Check sheet for the modelled part. Datum: model origin and axes. Units: mm. Face numbers are marked on the shaded views. Round coordinates to 2 decimals unless told otherwise and drop trailing zeros. Write each loop counter-clockwise with the first axis right and the second up, starting at its lowest first coordinate (ties: lowest second). Pieces come first, ordered by that corner, then holes.
Item 1: Material ranges on line 1 along X through (y, z) = (50.8, 11.75) (3 decimals); line 2 along Y through (x, z) = (1, 10.25); line 3 along X through (y, z) = (50, 2.25) (3 decimals), recorded low to high.
Item 2: Section check B-B, the plane x = 46. Record the cut outline in (y, z).
Item 3: Depth check by flat-ended pin: pin 1 (4 mm diameter, centred on y = -44.5, z = 3, fed in from -X); pin 2 (2 mm diameter, centred on x = 36, z = 6, fed in from +Y) (3 decimals); pin 3 (12 mm diameter, centred on y = 26, z = 4, fed in from -X); pin 4 (5.5 mm diameter, centred on x = 0, y = -63.5, fed in from +Z). Enter the tip coordinate at first touch or a pass-through.
Item 4: Section check D-D, the plane y = -38. Record the cut outline in (x, z) (3 decimals).
Item 5: Section check C-C, the plane x = 23. Record the cut outline in (y, z), plus the area to 3 significant figures.
Item 6: Section check A-A, the plane z = 19.5. State how many separate pieces and enclosed holes the cut face has, plus the area to 3 significant figures.
Item 7: Release check for a two-part mould opening along Y. For the marked faces 1, 2 and 3 record: pulls with the +Y half, pulls with the -Y half, needs draft (parallel to the pull), parting line crosses it, or undercut.
from build123d import *

# Parameters (mm, degrees)
F0_R     = 3.175
F1_DEPTH = 25.4


with BuildPart() as f1:
    # F0 (on Top) → F1 (new body)
    with BuildSketch(Plane.XY):
        with BuildLine():
            ThreePointArc((-9.525, 50.8), (-6.7351920908, 44.0648079092), (0, 41.275))
            ThreePointArc((0, 41.275), (6.7351920908, 44.0648079092), (9.525, 50.8))
            ThreePointArc((9.525, 50.8), (0, 60.325), (-9.525, 50.8))
        make_face()
        with BuildLine():
            ThreePointArc((3.175, 50.8), (2.2450640303, 48.5549359697), (0, 47.625))
            ThreePointArc((0, 47.625), (-2.2450640303, 53.0450640303), (3.175, 50.8))
        make_face(mode=Mode.SUBTRACT)
        with BuildLine():
            ThreePointArc((9.525, 50.8), (6.7351920908, 44.0648079092), (0, 41.275))
            Line((0, 41.275), (0, 36.5252))
            Line((0, 36.5252), (0, 15.875))
            ThreePointArc((0, 15.875), (9.7463072395, 12.5309664508), (15.3865384615, 3.9076923077))
            Line((15.3865384615, 3.9076923077), (9.525, 50.8))
        make_face()
        with BuildLine():
            Line((0, 36.5252), (0, 41.275))
            ThreePointArc((0, 41.275), (-6.7351920908, 44.0648079092), (-9.525, 50.8))
            Line((-9.525, 50.8), (-15.7474568951, 2.0082894055))
            ThreePointArc((-15.7474568951, 2.0082894055), (-10.4912828264, 11.9142188018), (0, 15.875))
            Line((0, 15.875), (0, 36.5252))
        make_face()
        with Locations((-3.175, 36.5252)):
            Circle(F0_R, mode=Mode.SUBTRACT)
        with BuildLine():
            ThreePointArc((15.3865384615, 3.9076923077), (9.7463072395, 12.5309664508), (0, 15.875))
            Line((0, 15.875), (0, 3.175))
            ThreePointArc((0, 3.175), (2.2450640303, 2.2450640303), (3.175, 0))
            ThreePointArc((3.175, 0), (2.2450640303, -2.2450640303), (0, -3.175))
            Line((0, -3.175), (0, -15.875))
            ThreePointArc((0, -15.875), (10.0526499203, -12.2865721249), (15.5606435644, -3.1435643564))
            Line((15.5606435644, -3.1435643564), (15.875, 0))
            Line((15.875, 0), (15.3865384615, 3.9076923077))
        make_face()
        with BuildLine():
            Line((0, 3.175), (0, 15.875))
            ThreePointArc((0, 15.875), (-10.4912828264, 11.9142188018), (-15.7474568951, 2.0082894055))
            ThreePointArc((-15.7474568951, 2.0082894055), (-11.9142188018, -10.4912828264), (0, -15.875))
            Line((0, -15.875), (0, -3.175))
            ThreePointArc((0, -3.175), (-3.175, 0), (0, 3.175))
        make_face()
        with BuildLine():
            ThreePointArc((0, -15.875), (-11.9142188018, -10.4912828264), (-15.7474568951, 2.0082894055))
            Line((-15.7474568951, 2.0082894055), (-16.0035761028, 0))
            Line((-16.0035761028, 0), (-9.525, -63.5))
            ThreePointArc((-9.525, -63.5), (-6.7351920908, -56.7648079092), (0, -53.975))
            Line((0, -53.975), (0, -15.875))
        make_face()
        with BuildLine():
            ThreePointArc((15.875, 0), (15.7524112928, 1.9690514116), (15.3865384615, 3.9076923077))
            Line((15.3865384615, 3.9076923077), (15.875, 0))
        make_face()
        with BuildLine():
            ThreePointArc((15.5606435644, -3.1435643564), (10.0526499203, -12.2865721249), (0, -15.875))
            Line((0, -15.875), (0, -53.975))
            Line((0, -53.975), (0.6794904459, -53.9992675159))
            ThreePointArc((0.6794904459, -53.9992675159), (6.9712901065, -57.0094885216), (9.525, -63.5))
            Line((9.525, -63.5), (36.5125, -63.5))
            ThreePointArc((36.5125, -63.5), (38.8373399243, -57.8873399243), (44.45, -55.5625))
            Line((44.45, -55.5625), (14.6753932646, -54.499121188))
            ThreePointArc((14.6753932646, -54.499121188), (11.8227843813, -53.1408361956), (10.8618983328, -50.1310166722))
            Line((10.8618983328, -50.1310166722), (15.5606435644, -3.1435643564))
        make_face()
        with BuildLine():
            ThreePointArc((15.5606435644, -3.1435643564), (15.7962153946, -1.5796215395), (15.875, 0))
            Line((15.875, 0), (15.5606435644, -3.1435643564))
        make_face()
        with BuildLine():
            Line((0, -60.325), (0, -53.975))
            ThreePointArc((0, -53.975), (-6.7351920908, -56.7648079092), (-9.525, -63.5))
            ThreePointArc((-9.525, -63.5), (-6.7351920908, -70.2351920908), (0, -73.025))
            Line((0, -73.025), (0.6794904459, -73.0007324841))
            ThreePointArc((0.6794904459, -73.0007324841), (6.9712901065, -69.9905114784), (9.525, -63.5))
            Line((9.525, -63.5), (3.175, -63.5))
            ThreePointArc((3.175, -63.5), (-2.2450640303, -65.7450640303), (0, -60.325))
        make_face()
        with BuildLine():
            Line((0.6794904459, -73.0007324841), (0, -73.025))
            ThreePointArc((0, -73.025), (0.3399618281, -73.0189311877), (0.6794904459, -73.0007324841))
        make_face()
        with BuildLine():
            Line((36.5125, -63.5), (9.525, -63.5))
            ThreePointArc((9.525, -63.5), (6.9712901065, -69.9905114784), (0.6794904459, -73.0007324841))
            Line((0.6794904459, -73.0007324841), (44.45, -71.4375))
            ThreePointArc((44.45, -71.4375), (38.8373399243, -69.1126600757), (36.5125, -63.5))
        make_face()
        with BuildLine():
            ThreePointArc((44.45, -55.5625), (38.8373399243, -57.8873399243), (36.5125, -63.5))
            Line((36.5125, -63.5), (41.275, -63.5))
            ThreePointArc((41.275, -63.5), (42.2049359697, -61.2549359697), (44.45, -60.325))
            Line((44.45, -60.325), (44.45, -55.5625))
        make_face()
        with BuildLine():
            Line((41.275, -63.5), (36.5125, -63.5))
            ThreePointArc((36.5125, -63.5), (38.8373399243, -69.1126600757), (44.45, -71.4375))
            Line((44.45, -71.4375), (44.45, -66.675))
            ThreePointArc((44.45, -66.675), (42.2049359697, -65.7450640303), (41.275, -63.5))
        make_face()
        with BuildLine():
            ThreePointArc((52.3875, -63.5), (50.0626600757, -57.8873399243), (44.45, -55.5625))
            Line((44.45, -55.5625), (44.45, -60.325))
            ThreePointArc((44.45, -60.325), (46.6950640303, -61.2549359697), (47.625, -63.5))
            ThreePointArc((47.625, -63.5), (46.6950640303, -65.7450640303), (44.45, -66.675))
            Line((44.45, -66.675), (44.45, -71.4375))
            ThreePointArc((44.45, -71.4375), (50.0626600757, -69.1126600757), (52.3875, -63.5))
        make_face()
        with BuildLine():
            Line((0.6794904459, -53.9992675159), (0, -53.975))
            Line((0, -53.975), (0, -60.325))
            ThreePointArc((0, -60.325), (2.2450640303, -61.2549359697), (3.175, -63.5))
            Line((3.175, -63.5), (9.525, -63.5))
            ThreePointArc((9.525, -63.5), (6.9712901065, -57.0094885216), (0.6794904459, -53.9992675159))
        make_face()
    extrude(amount=F1_DEPTH)


solid = f1.part
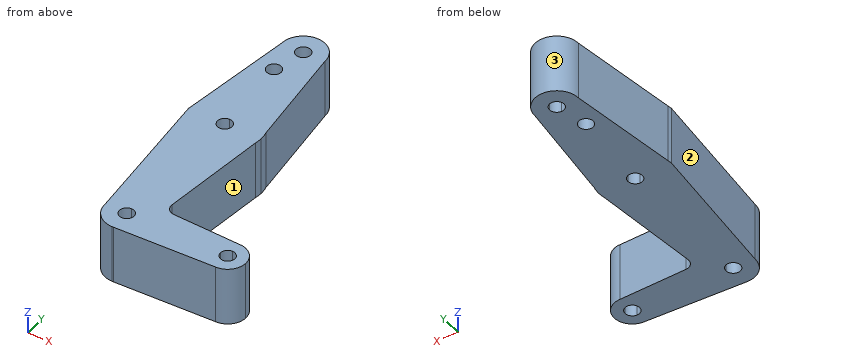
Values found:
1. line 1: x = -9.525 to -3.175, 3.175 to 9.525
1. line 2: y = -72.99 to -66.51, -60.49 to -3.01, 3.01 to 47.79, 53.81 to 60.27
1. line 3: x = -9.627 to -3.073, 3.073 to 9.625
2. outline: (-71.28, 0) - (-66.27, 0) - (-66.27, 25.4) - (-71.28, 25.4) - close; (-60.73, 0) - (-55.72, 0) - (-55.72, 25.4) - (-60.73, 25.4) - close
3. pin 1: stops at x = -11.67
3. pin 2: stops at y = -55.225
3. pin 3: stops at x = -13.45
3. pin 4: passes through
4. outline: (-12.127, 0) - (12.075, 0) - (12.075, 25.4) - (-12.127, 25.4) - close
5. outline: (-72.2, 0) - (-54.8, 0) - (-54.8, 25.4) - (-72.2, 25.4) - close
5. area: 442 mm2
6. separate pieces: 1
6. enclosed holes: 5
6. area: 3,750 mm2
7. face 1: undercut
7. face 2: pulls with the -Y half
7. face 3: pulls with the +Y half
